from build123d import *

# Parameters (mm, degrees)
F1_DEPTH = 3.175
F2_R     = 15.24


with BuildPart() as f1:
    # F0 (on Top) → F1 (new body)
    with BuildSketch(Plane.XY):
        with BuildLine():
            ThreePointArc((-0.7964807044, 11.0075218), (-0.3985002187, 11.0291031034), (0, 11.0363))
            Line((0, 11.0363), (0, 14.7955))
            ThreePointArc((0, 14.7955), (-3.1855144618, 15.2852623433), (-6.0767868514, 16.709310625))
            ThreePointArc((-6.0767868514, 16.709310625), (-7.9955151986, 15.8808103291), (-9.803769889, 14.832885625))
            ThreePointArc((-9.803769889, 14.832885625), (-5.6346854623, 12.132440692), (-0.7964807044, 11.0075218))
        make_face()
        with BuildLine():
            Line((0, 14.7955), (0, 11.0363))
            ThreePointArc((0, 11.0363), (0.3985002187, 11.0291031034), (0.7964807044, 11.0075218))
            ThreePointArc((0.7964807044, 11.0075218), (5.6346854623, 12.132440692), (9.803769889, 14.832885625))
            ThreePointArc((9.803769889, 14.832885625), (7.9955151986, 15.8808103291), (6.0767868514, 16.709310625))
            ThreePointArc((6.0767868514, 16.709310625), (3.1855144618, 15.2852623433), (0, 14.7955))
        make_face()
        with BuildLine():
            ThreePointArc((-9.9310338637, -4.8139883763), (-9.5577161638, 5.51815), (-0.7964807044, 11.0075218))
            ThreePointArc((-0.7964807044, 11.0075218), (-5.6346854623, 12.132440692), (-9.803769889, 14.832885625))
            ThreePointArc((-9.803769889, 14.832885625), (-15.3979316793, 8.89), (-17.7475407072, 1.0738709642))
            ThreePointArc((-17.7475407072, 1.0738709642), (-13.3243445803, -1.1864395933), (-9.9310338637, -4.8139883763))
        make_face()
        with BuildLine():
            ThreePointArc((9.803769889, 14.832885625), (5.6346854623, 12.132440692), (0.7964807044, 11.0075218))
            ThreePointArc((0.7964807044, 11.0075218), (8.0805358018, 7.5169713879), (11.0363, 0))
            ThreePointArc((11.0363, 0), (10.7564349745, -2.4696202805), (9.9310338637, -4.8139883763))
            ThreePointArc((9.9310338637, -4.8139883763), (13.3243445803, -1.1864395933), (17.7475407072, 1.0738709642))
            ThreePointArc((17.7475407072, 1.0738709642), (15.3979316793, 8.89), (9.803769889, 14.832885625))
        make_face()
        with BuildLine():
            ThreePointArc((-9.1345531593, -6.1935334237), (-9.5577161638, -5.51815), (-9.9310338637, -4.8139883763))
            ThreePointArc((-9.9310338637, -4.8139883763), (-13.3243445803, -1.1864395933), (-17.7475407072, 1.0738709642))
            ThreePointArc((-17.7475407072, 1.0738709642), (-17.750942777, -1.0160858862), (-17.5090809067, -3.0920035258))
            ThreePointArc((-17.5090809067, -3.0920035258), (-13.0514307386, -7.0051425696), (-11.3925452561, -12.7))
            ThreePointArc((-11.3925452561, -12.7), (-11.4024871162, -13.1590839469), (-11.4322940553, -13.6173070992))
            ThreePointArc((-11.4322940553, -13.6173070992), (-9.7554275784, -14.8647244429), (-7.9437708182, -15.9067565892))
            ThreePointArc((-7.9437708182, -15.9067565892), (-7.6731363163, -14.3135188044), (-7.5825452561, -12.7))
            ThreePointArc((-7.5825452561, -12.7), (-7.9759147279, -9.3554957079), (-9.1345531593, -6.1935334237))
        make_face()
        with BuildLine():
            ThreePointArc((14.4145, 25.4), (-5.7646061958, 38.6116284256), (-9.803769889, 14.832885625))
            ThreePointArc((-9.803769889, 14.832885625), (-7.9955151986, 15.8808103291), (-6.0767868514, 16.709310625))
            ThreePointArc((-6.0767868514, 16.709310625), (-4.8997007095, 34.8046984645), (10.6045, 25.4))
            ThreePointArc((10.6045, 25.4), (9.4046984645, 20.5002992905), (6.0767868514, 16.709310625))
            ThreePointArc((6.0767868514, 16.709310625), (7.9955151986, 15.8808103291), (9.803769889, 14.832885625))
            ThreePointArc((9.803769889, 14.832885625), (13.2116284256, 19.6353938042), (14.4145, 25.4))
        make_face()
        with BuildLine():
            ThreePointArc((9.1345531593, -6.1935334237), (0, -11.0363), (-9.1345531593, -6.1935334237))
            ThreePointArc((-9.1345531593, -6.1935334237), (-7.9759147279, -9.3554957079), (-7.5825452561, -12.7))
            ThreePointArc((-7.5825452561, -12.7), (-7.6731363163, -14.3135188044), (-7.9437708182, -15.9067565892))
            ThreePointArc((-7.9437708182, -15.9067565892), (0, -17.78), (7.9437708182, -15.9067565892))
            ThreePointArc((7.9437708182, -15.9067565892), (7.689659118, -10.9460010987), (9.1345531593, -6.1935334237))
        make_face()
        with BuildLine():
            ThreePointArc((-17.5090809067, -3.0920035258), (-17.750942777, -1.0160858862), (-17.7475407072, 1.0738709642))
            ThreePointArc((-17.7475407072, 1.0738709642), (-34.480368439, -19.90725), (-7.9437708182, -15.9067565892))
            ThreePointArc((-7.9437708182, -15.9067565892), (-9.7554275784, -14.8647244429), (-11.4322940553, -13.6173070992))
            ThreePointArc((-11.4322940553, -13.6173070992), (-31.1808116506, -18.00225), (-17.5090809067, -3.0920035258))
        make_face()
        with BuildLine():
            ThreePointArc((17.7475407072, 1.0738709642), (13.3243445803, -1.1864395933), (9.9310338637, -4.8139883763))
            ThreePointArc((9.9310338637, -4.8139883763), (9.5577161638, -5.51815), (9.1345531593, -6.1935334237))
            ThreePointArc((9.1345531593, -6.1935334237), (7.689659118, -10.9460010987), (7.9437708182, -15.9067565892))
            ThreePointArc((7.9437708182, -15.9067565892), (9.7554275784, -14.8647244429), (11.4322940553, -13.6173070992))
            ThreePointArc((11.4322940553, -13.6173070992), (12.8132788617, -7.39775), (17.5090809067, -3.0920035258))
            ThreePointArc((17.5090809067, -3.0920035258), (17.7121407306, -1.5519248499), (17.78, 0))
            ThreePointArc((17.78, 0), (17.7718833241, 0.5371807083), (17.7475407072, 1.0738709642))
        make_face()
        with BuildLine():
            ThreePointArc((36.4115452561, -12.7), (30.5563480002, -1.1018903788), (17.7475407072, 1.0738709642))
            ThreePointArc((17.7475407072, 1.0738709642), (17.7718833241, 0.5371807083), (17.78, 0))
            ThreePointArc((17.78, 0), (17.7121407306, -1.5519248499), (17.5090809067, -3.0920035258))
            ThreePointArc((17.5090809067, -3.0920035258), (27.6919026866, -3.7543854824), (32.6015452561, -12.7))
            ThreePointArc((32.6015452561, -12.7), (22.456129203, -23.2945581399), (11.4322940553, -13.6173070992))
            ThreePointArc((11.4322940553, -13.6173070992), (9.7554275784, -14.8647244429), (7.9437708182, -15.9067565892))
            ThreePointArc((7.9437708182, -15.9067565892), (23.6105640606, -27.0239089399), (36.4115452561, -12.7))
        make_face()
    extrude(amount=F1_DEPTH)

    # F2
    f2_edges = [f1.edges().sort_by_distance(p)[0] for p in [
        (-9.80377, 14.832886, 1.5875),
        (-17.747541, 1.073871, 1.5875),
        (-7.943771, -15.906757, 1.5875),
        (17.747541, 1.073871, 1.5875),
        (7.943771, -15.906757, 1.5875),
        (9.80377, 14.832886, 1.5875),
    ]]
    fillet(f2_edges, radius=F2_R)


solid = f1.part
The model under review builds one solid part; all positions refer to its coordinate system, in mm. Round coordinates to 2 decimals unless told otherwise and drop trailing zeros. Order: outer loops, then holes, each group sorted by start corner. A loop starts at its lowest first (then second) coordinate and runs counter-clockwise, first axis right, second up. Notation, with made-up numbers: (39, 60.25) -> (74, 60.25) arc R19 ccw to (74, 69.25) -> close; hole circle Ø2 at (-15.5, -4.5). An arc over 180 degrees is marked (long way). Write item = value, one per line. Start each with the question number.
Item 1: For line 1 along X through (y, z) = (-12.7, 1.2); line 2 along Y through (x, z) = (0, 0.8); line 3 along X through (y, z) = (-16, 0.8), list the stretches that pass through material, from the lowest coordinate up.
Item 2: Consider section A-A on x = 31. Write out the cut boundary in (y, z) (3 decimals), plus the area to 3 significant figures.
Item 3: Consider section B-B on z = 1.3. Count the separate pieces of the cut face and the enclosed holes in it, plus the area to 3 significant figures.
Item 4: Clearance check with flat-ended pins moving along their axes: pin 1 Ø1 at (x, z) = (4.5, 2.5) entering from -Y; pin 2 Ø6 at (x, y) = (3.5, -6) entering from -Z. State where each tip first meets the part, or that it passes through.
Conclusion:
q1.line_1 = -36.41 to -32.6, -11.39 to 11.39, 32.6 to 36.41
q1.line_2 = -17.78 to -11.04, 11.04 to 14.8, 36 to 39.81
q1.line_3 = -36.03 to -32.08, -11.92 to 11.92, 32.08 to 36.03
q2.outline = (-23.957, 0) -> (-18.304, 0) -> (-18.304, 3.175) -> (-23.957, 3.175) -> close; (-7.096, 0) -> (-1.443, 0) -> (-1.443, 3.175) -> (-7.096, 3.175) -> close
q2.area = 35.9 mm2
q3.separate_pieces = 1
q3.enclosed_holes = 4
q3.area = 1,320 mm2
q4.pin_1 = -18.49
q4.pin_2 = through
